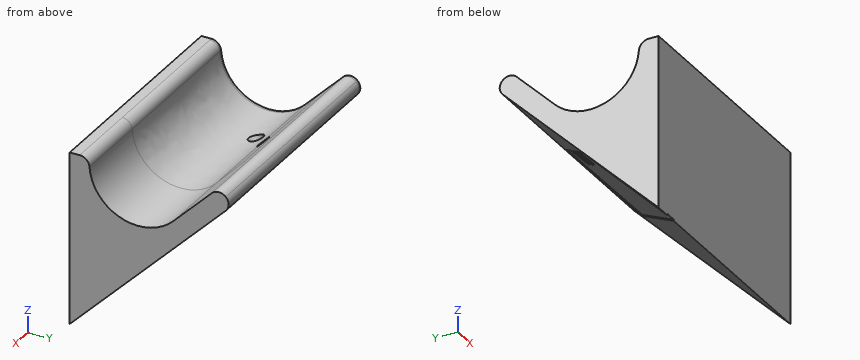
Autodesk Inventor part; units mm, degrees
ref_plane "Work Plane2" through (19.0401, 0, -19) normal (-1, 0, 0) x (0, 0, 1)
ref_plane "Work Plane3" through (19.0401, 18.7838, 5.4407) normal (0, -0.7071068, 0.7071068) x (1, 0, 0)
ref_plane "Work Plane4" through (66.9063, -11.5314, 4.4686) normal (1, 0, 0) x (0, 0, -1)
sketch "Sketch1" plane through (0, 0, 0) normal (1, 0, 0) x (0, 1, 0)
  line L0 (0, 0) -> (0, -19)
  line L1 (0, -19) -> (19, 0)
  line L2 (0, -19) -> (9.9437, -19) construction
  line L3 (0, -19) -> (19, 0)
  line L4 (19, 0) -> (0, 0)
  dimension "d0" = 19
  dimension "d1" = 45
extrude "Extrusion1" add sketch "Sketch1" along normal blind 61
sketch "Sketch2" plane through (61, 19, 0) normal (0, 0.7071068, -0.7071068) x (-1, 0, 0)
  line L0 (47, 0) -> (15, 0)
  line L1 (61, -26.8701) -> (0, -26.8701)
  line L2 (61, -26.8701) -> (0, -26.8701)
  line L3 (61, 0) -> (0, 0)
  line L4 (47, 0) -> (61, 0)
  line L5 (61, -26.8701) -> (61, 0)
  line L6 (61, 0) -> (61, -26.8701)
  line L7 (0, -26.8701) -> (0, 0)
  line L8 (0, 0) -> (0, -26.8701)
  line L9 (15, 0) -> (0, -26.8701)
  line L10 (47, 0) -> (61, -26.8701)
  point P0 (31, 0)
  point P1 (31, 0)
  dimension "d4" = 32
sketch "Sketch3" plane through (0, 0, 0) normal (-1, 0, 0) x (0, 0, 1)
  line L0 (-19, 0) -> (0, 19)
  line L1 (0, 19) -> (-12.7279, 6.2721)
  line L2 (-12.7279, 6.2721) -> (-9.8995, 3.4437)
  line L3 (-9.8995, 3.4437) -> (0, 13.3431)
  line L4 (0, 19) -> (0, 0)
  line L5 (-9.8995, 3.4437) -> (0, 3.4437)
  dimension "d5" = 18
  dimension "d6" = 4
extrude "Extrusion2" cut sketch "Sketch3" against normal blind 62 contours L3 L4 L5
sketch "Sketch4" plane through (61, 0, -19) normal (0, 0.7071068, -0.7071068) x (-1, 0, 0)
  line L0 (61, 26.8701) -> (0, 26.8701) construction
  line L1 (30.5, 26.8701) -> (30.5, 0) construction
  line L2 (61, 0) -> (0, 0) construction
  line L3 (30.5, 17.2) -> (30.5, -1.6) construction
  line L4 (52.0668, -4.3668) -> (8.9332, 38.7668) construction
  line L5 (41.9599, 0) -> (41.9599, -16.3079)
  line L6 (41.9599, -16.3079) -> (-10.9063, -16.3079)
  line L7 (-10.9063, -16.3079) -> (-10.9063, 26.8701)
  line L8 (17.1357, 30.5643) -> (-10.9063, 30.5643)
  line L9 (-10.9063, 30.5643) -> (-10.9063, 26.8701)
  line L10 (17.1357, 30.5643) -> (41.9599, 30.5643)
  line L11 (41.9599, 0) -> (41.9599, 30.5643)
  line L12 (36.9964, -16.3079) -> (-5.0421, 25.7306)
  line L13 (-5.0421, 25.7306) -> (19.4362, 28.5467)
  line L14 (19.4362, 28.5467) -> (27.1412, 20.8416)
  line L15 (27.1412, 20.8416) -> (25.4088, 19.1092)
  arc A0 (25.4088, 19.1092) -> (27.6009, 16.9172) centre (26.5048, 18.0132) ccw
  line L16 (27.6009, 16.9172) -> (29.3333, 18.6496)
  line L17 (39.262, -16.3307) -> (41.8467, 6.1362)
  line L18 (29.3333, 18.6496) -> (31.9496, 16.0333)
  line L19 (31.9496, 16.0333) -> (30.2172, 14.3009)
  arc A1 (30.2172, 14.3009) -> (32.4092, 12.1088) centre (31.3132, 13.2048) ccw
  line L20 (32.4092, 12.1088) -> (34.1416, 13.8412)
  line L21 (34.1416, 13.8412) -> (41.8467, 6.1362)
  line L22 (29.1919, 18.5081) -> (29.3333, 18.6496)
  line L23 (29.3333, 18.6496) -> (29.4747, 18.5081)
  point P0 (61, 13.435)
  point P1 (47, 26.8701)
  point P2 (15, 26.8701)
  dimension "d13" = 18.8
  dimension "d14" = 1.6
extrude "Extrusion4" cut sketch "Sketch2" against normal blind 62 contours L3 L5 L10 | L9 L7 L3
sketch "Sketch5" plane through (61, 0, -19) normal (0, 0.7071068, -0.7071068) x (-1, 0, 0)
  point P0 (61, 13.435)
extrude "Extrusion5" add sketch "Sketch4" against normal up to surface (4 mm away)
sketch "Sketch6" plane through (19.0401, 0, -19) normal (-1, 0, 0) x (0, 0, 1)
  line L0 (-11.5314, -11.5314) -> (-5.8745, -11.5314)
  line L1 (5.6569, 0) -> (-5.8745, -11.5314)
  line L2 (-11.5314, -11.5314) -> (0, 0)
  line L3 (21.6122, 21.6122) -> (-11.5314, -11.5314)
  line L4 (19, 0) -> (0, 0)
  line L5 (5.6569, 0) -> (0, 0)
  line L6 (-11.5314, -11.5314) -> (-8.703, -14.3598)
  line L7 (-11.5314, -11.5314) -> (-8.703, -14.3598)
  line L8 (-8.703, -14.3598) -> (-5.8745, -11.5314)
extrude "Extrusion6" cut sketch "Sketch6" against normal blind 62 contours L0 L8 L6
ref_plane "Work Plane2" through (19.0401, 0, -19) normal (-1, 0, 0) x (0, 0, 1)
split "Split1" plane through (19.0401, 0, -19) removes the side toward (-1, 0, 0)
ref_plane "Work Plane3" through (19.0401, 18.7838, 5.4407) normal (0, -0.7071068, 0.7071068) x (1, 0, 0)
split "Split2" plane through (19.0401, 18.7838, 5.4407) removes the side toward (0, -0.7071068, 0.7071068)
sketch "Sketch7" plane through (19.0401, -11.5314, -30.5314) normal (-1, 0, 0) x (0, 0, 1)
  line L0 (5.6569, 0) -> (0, 0)
  line L1 (0, 0) -> (35, 0)
  line L2 (35, 0) -> (35, 4)
  line L3 (35, 4) -> (4, 4)
  line L4 (0, 0) -> (33.1436, 33.1436)
  line L5 (4, 4) -> (0, 0)
  point P0 (30.5314, 11.5314)
  dimension "d29" = 35
  dimension "d30" = 4
extrude "Extrusion7" add sketch "Sketch7" against normal up to surface (52.8662 mm away)
sketch "Sketch8" plane through (71.9063, 21.6122, 2.6122) normal (0, 0.7071068, -0.7071068) x (-1, 0, 0)
  line L0 (30.3425, -2.0177) -> (38.0475, -9.7227)
  line L1 (62.973, -34.9311) -> (19.8395, 8.2024) construction
  line L2 (38.0475, -9.7227) -> (36.3151, -11.4551)
  arc A0 (36.3151, -11.4551) -> (38.5071, -13.6472) centre (37.4111, -12.5511) ccw
  line L3 (38.5071, -13.6472) -> (40.2395, -11.9147)
  line L4 (40.2395, -11.9147) -> (42.8558, -14.531)
  line L5 (42.8558, -14.531) -> (41.1234, -16.2635)
  arc A1 (41.1234, -16.2635) -> (43.3155, -18.4555) centre (42.2194, -17.3595) ccw
  line L6 (43.3155, -18.4555) -> (45.0479, -16.7231)
  line L7 (45.0479, -16.7231) -> (52.7529, -24.4281)
  line L8 (50.1709, -46.8722) -> (52.7529, -24.4281)
  line L9 (47.9026, -46.8722) -> (5.8642, -4.8337)
  line L10 (5.8642, -4.8337) -> (30.3425, -2.0177)
  line L11 (52.8662, -46.8722) -> (0, -46.8722)
  point P0 (71.9063, -17.1293)
extrude "Extrusion8" cut sketch "Sketch8" against normal blind 0.2
fillet "Fillet1" radius 10 1 edges at (45.4732, -7.5314, -20.8745)
fillet "Fillet1" radius 2 3 edges at (45.4732, -7.5314, 4.4686) (45.4732, 18.7838, 5.4407) (45.4732, 21.6122, 2.6122)
sketch "Sketch9" plane through (71.9063, -11.5314, -30.5314) normal (0, 0.7071068, -0.7071068) x (-1, 0, 0)
  arc A0 (36.3151, 35.417) -> (38.5071, 33.225) centre (37.4111, 34.321) ccw
  point P0 (71.9063, 29.7429)
hole "Hole1" at (34.4952, 12.7372, -6.2628) direction (0, -0.7071068, 0.7071068) diameter 2.85 end through all
sketch "Sketch10" plane through (71.9063, -11.5314, -30.5314) normal (0, 0.7071068, -0.7071068) x (-1, 0, 0)
  arc A0 (41.1234, 30.6087) -> (43.3155, 28.4167) centre (42.2194, 29.5127) ccw
  point P0 (71.9063, 29.7429)
hole "Hole2" at (29.6868, 9.3372, -9.6628) direction (0, -0.7071068, 0.7071068) diameter 2.85 end through all
ref_plane "Work Plane4" through (66.9063, -11.5314, 4.4686) normal (1, 0, 0) x (0, 0, -1)
split "Split3" plane through (66.9063, -11.5314, 4.4686) removes the side toward (1, 0, 0)
sketch "Sketch11" plane through (19.0401, -11.5314, -30.5314) normal (-1, 0, 0) x (0, 0, 1)
  arc A0 (34.5578, 28.901) -> (31.7294, 31.7294) centre (33.1436, 30.3152) ccw
  line L0 (0, 0) -> (31.7294, 31.7294)
  line L1 (0, 0) -> (35, 0)
  line L2 (35, 0) -> (35, 2.0266)
  arc A1 (35, 2.0266) -> (33.1332, 4.0222) centre (33, 2.0266) ccw
  arc A2 (26.7279, 21.0711) -> (33.1332, 4.0222) centre (33.799, 14) ccw
  line L3 (26.7279, 21.0711) -> (34.5578, 28.901)
  point P0 (30.5314, 11.5314)
extrude "Extrusion9" add sketch "Sketch11" along normal blind 0.5
properties part number "cutter" material "PET Plastic"
The listing builds one solid part. Answer for the finished solid, in the listing's coordinates (mm). Give positions to 0.01 mm unless a question says otherwise; leave off trailing zeros. Loops run counter-clockwise (first coordinate to the right, second up) from the corner with the lowest first, then second, coordinate; pieces in that order, holes last. Notation, with made-up numbers: M 42.25,18 L 100.25,18 A8 cw 100.25,32 Z; hole C 50.5,42 d4. An arc over 180 degrees is marked long. One line per item, written item: value.
1. Section B-B on z = -28 is taken. Determine the outline of the cut face in (x, y), plus the area to 3 significant figures.
Found:
outline: M 18.54,-11.53 L 66.91,-11.53 L 66.91,-9 L 27.58,-9 L 27.38,-9.29 L 21.35,-9.29 L 21.32,-9 L 18.54,-9 Z
area: 121 mm^2
2. Section A-A on z = -22 is taken. Determine the outline of the cut face in (x, y), plus the area to 3 significant figures.
Found:
outline: M 18.54,-11.53 L 66.91,-11.53 L 66.91,-3 L 36.07,-3 L 35.87,-3.29 L 20.37,-3.29 L 20.35,-3 L 18.54,-3 Z
area: 408 mm^2
3. Find the intervals of material crossed by probe 1 along X at (y, z) = (12, -6.5); probe 2 along Y at (x, z) = (24.5, 1); probe 3 along Z at (x, y) = (57.5, -6.5), in increasing order.
Found:
probe 1: 18.54 to 33.25, 35.74 to 66.91
probe 2: -11.53 to -7.27, 14.34 to 20
probe 3: -25.5 to -1.16
4. Each of these flat-tipped pins is pushed along its axis until it touches: P1, Ø10, axis at x = 47, y = 16, coming from the -Z side; P2, Ø3, axis at y = -3, z = -2, coming from the -X side; P3, Ø8, axis at x = 44, z = -7.5, coming from the +Y side; P4, Ø12, axis at x = 52.5, z = -22, coming from the +Y side. Where does it stop, or does it pass through?
Found:
P1: z = -7.71
P2: through
P3: y = 15.21
P4: y = 3
